Autodesk Inventor part; units mm, degrees
ref_plane "YZ Plane" through (0, 0, 0) normal (1, 0, 0) x (0, 1, 0)
sketch "Sketch1" plane through (0, 0, 0) normal (0, 0, 1) x (1, 0, 0)
  line L0 (0, 71.9938) -> (0, -26.8156)
  line L1 (-40.64, 0) -> (110.49, 0)
  line L2 (-19.05, 0) -> (-19.05, 57.8782)
  line L3 (24.13, 57.8782) -> (24.13, 39.5859)
  line L4 (-19.05, 0) -> (88.9, 0)
  line L5 (88.9, 0) -> (88.9, 25.4)
  line L6 (0, 41.1734) -> (24.13, 41.1734) construction
  line L7 (12.6388, 39.5859) -> (24.13, 39.5859)
  line L8 (24.13, 39.5859) -> (24.13, 42.7577)
  line L9 (24.13, 42.7577) -> (12.6392, 42.7577)
  line L10 (4.9628, 39.5889) -> (24.13, 42.7577) construction
  line L11 (24.13, 39.5859) -> (4.9638, 42.7609) construction
  line L12 (39.9796, 0) -> (88.9, 0) construction
  line L13 (88.9, 0) -> (88.9, -12.7) construction
  line L14 (88.9, -12.7) -> (39.9796, -12.7) construction
  line L15 (39.9796, -12.7) -> (39.9796, 0) construction
  line L16 (52.6796, -12.7) -> (52.6796, 0) construction
  line L17 (78.0796, -12.7) -> (78.0796, 0) construction
  line L18 (38.3159, 25.4) -> (88.9, 25.4)
  line L19 (16.8601, 41.1734) -> (16.8601, 57.8782) construction
  line L20 (12.7635, 41.1734) -> (12.7635, 34.371) construction
  line L21 (24.13, 39.5859) -> (38.3159, 25.4)
  line L22 (-19.05, 57.8782) -> (24.13, 57.8782)
  arc A0 (12.6392, 42.7577) -> (12.6388, 39.5859) centre (0, 41.1734) ccw
  point P0 (14.5469, 41.1734)
  dimension "d1" = 41.1734
  dimension "d3" = 107.95
  dimension "d4" = 25.4
  dimension "d7" = 24.13
  dimension "d13" = 19.05
  dimension "d15" = 39.9796
  dimension "d16" = 0
  dimension "d17" = 12.7
  dimension "d18" = 12.7
  dimension "d19" = 25.4
  dimension "d20" = 52.6796
  dimension "d39" = 16.8601
  dimension "d49" = 135
  dimension "d75" = 12.7381
extrude "Extrusion1" add sketch "Sketch1" along normal mid plane 17.78 contours L22 L3 L9 A0 L0 | L0 A0 L1 L2 L22 | A0 L7 L21 L18 L5 L1 L0
ref_plane "Work Plane1" through (0, 50.8, 0) normal (0, 1, 0) x (-1, 0, 0)
sketch "Sketch2" plane through (0, 50.8, 0) normal (0, 1, 0) x (-1, 0, 0)
  line L0 (0, -7.112) -> (0, 7.112)
  line L1 (-97.8865, 0) -> (16.3144, 0)
  line L2 (-56.1721, 5.08) -> (-49.1871, 5.08)
  line L3 (-49.1871, 5.08) -> (-49.1871, -5.08)
  line L4 (-49.1871, -5.08) -> (-56.1721, -5.08)
  line L5 (-56.1721, -5.08) -> (-56.1721, 5.08)
  line L6 (-56.1721, 5.08) -> (-49.1871, -5.08) construction
  line L7 (-49.1871, 5.08) -> (-56.1721, -5.08) construction
  line L8 (-81.5721, 5.08) -> (-74.5871, 5.08)
  line L9 (-74.5871, 5.08) -> (-74.5871, -5.08)
  line L10 (-74.5871, -5.08) -> (-81.5721, -5.08)
  line L11 (-81.5721, -5.08) -> (-81.5721, 5.08)
  line L12 (-81.5721, 5.08) -> (-74.5871, -5.08) construction
  line L13 (-74.5871, 5.08) -> (-81.5721, -5.08) construction
  point P0 (0, 0)
  point P1 (-52.6796, 0)
  point P2 (-78.0796, 0)
  dimension "d22" = 52.6796
  dimension "d23" = 25.4
  dimension "d24" = 10.16
  dimension "d25" = 6.985
extrude "Extrusion2" cut sketch "Sketch2" against normal up to next
sketch "Sketch3" plane through (0, 0, 0) normal (0, 0, 1) x (1, 0, 0)
  point P0 (0, 0)
fillet "Fillet1" radius 3.175 8 edges at (49.1871, 12.7, -5.08) (56.1721, 12.7, -5.08) (56.1721, 12.7, 5.08) (49.1871, 12.7, 5.08) (74.5871, 12.7, 5.08) (74.5871, 12.7, -5.08) (81.5721, 12.7, -5.08) (81.5721, 12.7, 5.08)
sketch "Sketch4" plane through (-19.05, 57.8782, 8.89) normal (0, 1, 0) x (1, 0, 0)
  line L0 (129.5216, 7.8564) -> (-21.59, 9.525)
  line L1 (43.18, 19.05) -> (43.18, 0)
  line L2 (19.05, 22.86) -> (19.05, -3.81)
  line L3 (116.9365, 8.89) -> (2.7356, 8.89)
  point P0 (19.05, 9.525)
  point P1 (129.5216, 7.8564)
  point P2 (-21.59, 9.525)
  point P3 (35.9156, 8.89)
  dimension "d38" = 16.8656
  dimension "d79" = 0
sketch "Sketch5" plane through (-19.05, 57.8782, 8.89) normal (0, 1, 0) x (1, 0, 0)
  point P0 (19.05, 9.525)
hole "Hole2" at (16.8656, 57.8782, 0) direction (0, -1, 0) diameter 5.4102 end up to surface counterbore diameter 10.541 counterbore depth 6.35
chamfer "Chamfer1" distance 25.4 angle 45 1 edges at (-19.05, 0, 0)
sketch "Sketch6" plane through (0, 0, 0) normal (1, 0, 0) x (0, 1, 0)
  line L0 (41.1734, -12.446) -> (41.1734, 12.446)
  line L1 (-11.5756, 0) -> (69.4538, 0)
  line L2 (28.4353, -4.7625) -> (28.1813, -4.7625)
  line L3 (28.1813, -4.7625) -> (28.1813, 4.7625)
  line L4 (28.1813, 4.7625) -> (28.4353, 4.7625)
  line L5 (28.4353, 4.7625) -> (28.4353, -4.7625)
  line L6 (28.4353, -4.7625) -> (28.1813, 4.7625) construction
  line L7 (28.1813, -4.7625) -> (28.4353, 4.7625) construction
  line L8 (28.4353, 8.89) -> (28.4353, -8.89)
  line L9 (57.8782, -8.89) -> (42.7577, -8.89)
  line L10 (42.7577, 8.89) -> (57.8782, 8.89)
  point P0 (0, 0)
  point P1 (28.3083, 0)
  dimension "d53" = 0
  dimension "d54" = 9.525
  dimension "d55" = 0.254
  dimension "d56" = 17.78
revolve "Revolution1" [suppressed]
hole "Hole3" at (16.8656, 39.5859, 0) direction (0, -1, 0) diameter 4.1402 depth 14.1986 tip angle 118
fillet "Fillet2" radius 0.254 2 edges at (12.6392, 42.7577, 0) (12.6388, 39.5859, 0)
fillet "Fillet3" radius 0.635 1 edges at (24.13, 57.8782, 0)
fillet "Fillet4" radius 3.175 5 edges at (-19.05, 57.8782, 0) (-19.05, 25.4, 0) (6.35, 0, 0) (88.9, 25.4, 0) (88.9, 0, 0)
chamfer "Chamfer2" [suppressed]
fillet "Fillet5" radius 3.175 1 edges at (38.3159, 25.4, 0)
properties part number "J005363" material "ALUMINUM, 6061-T651"
Here's how the part is built. I have some questions about the finished solid (model axes, mm). A direction names the side the tool comes from. Give positions to 0.01 mm unless a question says otherwise; leave off trailing zeros. Order: outer loops, then holes, each group sorted by start corner. A loop starts at its lowest first (then second) coordinate and runs counter-clockwise, first axis right, second up. Notation, with made-up numbers: M 17.5,34.5 L 72.5,34.5 A24 cw 72.5,44.5 Z; hole C 70,58 d1. An arc over 180 degrees is marked long. Answer as a JSON object with one key per item and string values. Group by question number.
1) Suppose I cut it at D-D, the plane x = 55. Write out the boundary of the cut face in (y, z), plus the area to 3 significant figures.
2) Suppose I cut it at A-A, the plane y = 16.5. Write out the boundary of the cut face in (x, z) (3 decimals).
3) On a 3-axis mill with a long thin cutter (end or side, diameter ignored), from which of +Z, -Z, +X, -X, +Y, -Y can I reach the whole of each face in a straight line? I mean faces 1 (the flat face through (81.572, 13, 0)), 2 (the cylindrical face through (19.506, 47.082, -0.586)), 3 (the flat face through (62, 25.4, 0)), 4 (the flat face through (20, 42.758, 0)). Say none if no direction works.
4) Please list where these lines run through material, in increasing order: L1, parallel to X at y = 5.5, z = -2; L2, parallel to X at y = 23, z = 0.5; L3, parallel to X at y = 50.5, z = 6.75. Write a range as [from, to].
5) We'd pull the mould along Z, two halves only. Please class faces 5 (the cylindrical face through (80.62, 12.52, -4.17)), 6 (the cylindrical face through (6.43, 0.25, 0.12)): pulls with the +Z half, pulls with the -Z half, needs draft (parallel to the pull), parting line crosses it, or undercut.
6) I'm going to push flat-ended pins straight in: pin 1 Ø3.5 at (x, z) = (17, 2.5) entering from +Y; pin 2 Ø1.1 at (y, z) = (12.5, 0.5) entering from -X; pin 3 Ø3 at (x, z) = (55.5, 3) entering from +Y. Where does each tip first touch, or does it pass through?
7) Suppose I cut it at B-B, the plane x = 0. Write out the boundary of the cut face in (y, z).
Results found:
{
 "1": {"outline": "M 0,-8.89 L 25.4,-8.89 L 25.4,-4.37 L 0,-4.37 Z; M 0,4.37 L 25.4,4.37 L 25.4,8.89 L 0,8.89 Z", "area": "230 mm²"},
 "2": {"outline": "M -10.15,-8.89 L 88.9,-8.89 L 88.9,8.89 L -10.15,8.89 Z; hole M 49.187,-1.905 A3.175 ccw 52.362,-5.08 L 52.997,-5.08 A3.175 ccw 56.172,-1.905 L 56.172,1.905 A3.175 ccw 52.997,5.08 L 52.362,5.08 A3.175 ccw 49.187,1.905 Z; hole M 74.587,-1.905 A3.175 ccw 77.762,-5.08 L 78.397,-5.08 A3.175 ccw 81.572,-1.905 L 81.572,1.905 A3.175 ccw 78.397,5.08 L 77.762,5.08 A3.175 ccw 74.587,1.905 Z"},
 "3": {"face 1": "+Y, -Y", "face 2": "+Y", "face 3": "+Z, -Z, +X, +Y", "face 4": "+Z, -Z, +X"},
 "4": {"L1": "[0.85, 49.19], [56.17, 74.59], [81.57, 88.9]", "L2": "[-16.65, 49.19], [56.17, 74.59], [81.57, 88.8]", "L3": "[-19.05, -8.68], [8.68, 24.13]"},
 "5": {"face 5": "undercut", "face 6": "needs draft"},
 "6": {"pin 1": "y = 51.53", "pin 2": "x = -6.7", "pin 3": "y = 25.4"},
 "7": {"outline": "M 6.35,-8.89 L 28.44,-8.89 L 28.44,8.89 L 6.35,8.89 Z; M 53.91,-8.89 L 57.88,-8.89 L 57.88,8.89 L 53.91,8.89 Z"}
}
